For this review, take the finished solid that the model builds, in its own axes (mm). Round coordinates to 2 decimals unless told otherwise and drop trailing zeros. Write each loop counter-clockwise with the first axis right and the second up, starting at its lowest first coordinate (ties: lowest second). Pieces come first, ordered by that corner, then holes. Notation, with made-up numbers: (15, 13.25) -> (19, 13.25) arc R18 ccw to (19, 17.25) -> close; hole circle Ø3 at (10, 71.25). An arc over 180 degrees is marked (long way). Answer in a Markdown table with one row per item. Add a question column.
```python
from build123d import *

# Parameters (mm, degrees)
SKETCH1_R           = 57.5
SKETCH1_R_2         = 40.6
BOSS_EXTRUDE1_DEPTH = 3
FILLET1_R           = 10
SKETCH2_R           = 2.6
SKETCH2_R_2         = 12.5
CUT_EXTRUDE1_DEPTH  = 4


with BuildPart() as part:
    # Sketch1 → Boss-Extrude1 (new body)
    with BuildSketch(Plane(origin=(0, 0, 0), x_dir=(1, 0, 0), z_dir=(0, 1, 0))):
        with BuildLine():
            Line((170, 57.5), (0, 57.5))
            ThreePointArc((0, 57.5), (40.658639918, 40.658639918), (57.5, 0))
            ThreePointArc((57.5, 0), (40.658639918, -40.658639918), (0, -57.5))
            Line((0, -57.5), (170, -57.5))
            Line((170, -57.5), (170, 57.5))
        make_face()
        Circle(SKETCH1_R)
        Circle(SKETCH1_R_2, mode=Mode.SUBTRACT)
    extrude(amount=BOSS_EXTRUDE1_DEPTH)

    # Fillet1
    fillet1_edges = [part.edges().sort_by_distance(p)[0] for p in [
        (170, 1.5, -57.5),
        (170, 1.5, 57.5),
    ]]
    fillet(fillet1_edges, radius=FILLET1_R)

    # Sketch2 → Cut-Extrude1 (cut, through all)
    with BuildSketch(Plane(origin=(0, 3, 0), x_dir=(1, 0, 0), z_dir=(0, 1, 0))):
        with Locations((160, 47.5)):
            Circle(SKETCH2_R)
        with Locations((160, -47.5)):
            Circle(SKETCH2_R)
        with Locations((30, -47.5)):
            Circle(SKETCH2_R)
        with Locations((30, 47.5)):
            Circle(SKETCH2_R)
        with Locations((65, 0)):
            Circle(SKETCH2_R_2)
    extrude(amount=-CUT_EXTRUDE1_DEPTH, mode=Mode.SUBTRACT)


solid = part.part
```
1. Clearance check with flat-ended pins moving along their axes: pin 1 Ø6 at (x, z) = (30, 47.5) entering from -Y; pin 2 Ø1 at (y, z) = (2, -42) entering from -X; pin 3 Ø4 at (x, z) = (30, -47.5) entering from +Y. State where each tip first meets the part, or that it passes through.
2. We need section C-C (z = -4.5). Write out the cut boundary in (x, y), plus the area to 3 significant figures.
3. For L1, parallel to X at y = 1.45, z = 0; L2, parallel to Z at x = 66, y = 0.3; L3, parallel to Z at x = 0, y = 1.1, list the stretches that pass through material, from the lowest coordinate up. Write a range as [from, to].
4. The part is to be moulded in two halves that separate along Z. For faces 1 (the cylindrical face through (166.99, 1.52, -54.65)), 2 (the cylindrical face through (-32.22, 1.48, 24.7)), 3 (the cylindrical face through (167.15, 1.52, 54.49)), 4 (the cylindrical face through (162.4, 1.5, -46.5)), say which applies: pulls with the +Z half, pulls with the -Z half, needs draft (parallel to the pull), parting line crosses it, or undercut.
5. We need section B-B (x = 65). Write out the cut boundary in (y, z).
6. We need section D-D (z = -33.5). Write out the cut boundary in (x, y).
7. We need section A-A (y = 1.75). Write out the cut boundary in (x, z), plus the area to 3 significant figures.
Response:
| question | item | result |
|---|---|---|
| 1 | pin 1 | y = 0 |
| 1 | pin 2 | x = -39.8 |
| 1 | pin 3 | through |
| 2 | outline | (-57.32, 0) -> (-40.35, 0) -> (-40.35, 3) -> (-57.32, 3) -> close; (40.35, 0) -> (53.34, 0) -> (53.34, 3) -> (40.35, 3) -> close; (76.66, 0) -> (170, 0) -> (170, 3) -> (76.66, 3) -> close |
| 2 | area | 370 mm2 |
| 3 | L1 | [-57.5, -40.6], [40.6, 52.5], [77.5, 170] |
| 3 | L2 | [-57.5, -12.46], [12.46, 57.5] |
| 3 | L3 | [-57.5, -40.6], [40.6, 57.5] |
| 4 | face 1 | pulls with the -Z half |
| 4 | face 2 | undercut |
| 4 | face 3 | pulls with the +Z half |
| 4 | face 4 | undercut |
| 5 | outline | (0, -57.5) -> (3, -57.5) -> (3, -12.5) -> (0, -12.5) -> close; (0, 12.5) -> (3, 12.5) -> (3, 57.5) -> (0, 57.5) -> close |
| 6 | outline | (-46.73, 0) -> (-22.94, 0) -> (-22.94, 3) -> (-46.73, 3) -> close; (22.94, 0) -> (170, 0) -> (170, 3) -> (22.94, 3) -> close |
| 7 | outline | (0, -57.5) -> (160, -57.5) arc R10 ccw to (170, -47.5) -> (170, 47.5) arc R10 ccw to (160, 57.5) -> (0, 57.5) arc R57.5 ccw to start; hole circle Ø81.2 at (0, 0); hole circle Ø5.2 at (30, -47.5); hole circle Ø5.2 at (30, 47.5); hole circle Ø25 at (65, 0); hole circle Ø5.2 at (160, -47.5); hole circle Ø5.2 at (160, 47.5) |
| 7 | area | 18,900 mm2 |
